Design review of the part shown in the three views and the two pictorial views. Dimensions are in mm from the part's minimum x, y and z. A direction names the side the tool comes from. Give positions to 0.01 mm unless a question says otherwise; leave off trailing zeros. Order: outer loops, then holes, each group sorted by start corner. A loop starts at its lowest first (then second) coordinate and runs counter-clockwise, first axis right, second up.
Item 1: Consider section C-C (z = 156.5). Give the boundary of the cut face in (x, y).
Item 2: Machinability: for the marked faces 1, 2 and 3, which of the approach directions +Z, -Z, +X, -X, +Y, -Y give a long, thin tool a straight path to every point of the face, cutting with its end or side? Answer none if there is none.
Item 3: For probe 1 along Z at (x, y) = (27, 58.5); probe 2 along X at (y, z) = (32.5, 111); probe 3 along Y at (x, z) = (31.5, 153.5), list the stretches that pass through material, from the lowest coordinate up.
Item 4: Consider section A-A (y = 32.25). Give the boundary of the cut face in (x, z).
Item 5: For P1, Ø8, axis at y = 23.5, z = 147.5, coming from the -X side; P2, Ø10, axis at y = 51.5, z = 87.5, coming from the -X side; P3, Ø4, axis at y = 41, z = 140, coming from the -X side, all flat-tipped, find the tip position at first contact; note any pin that passes through.
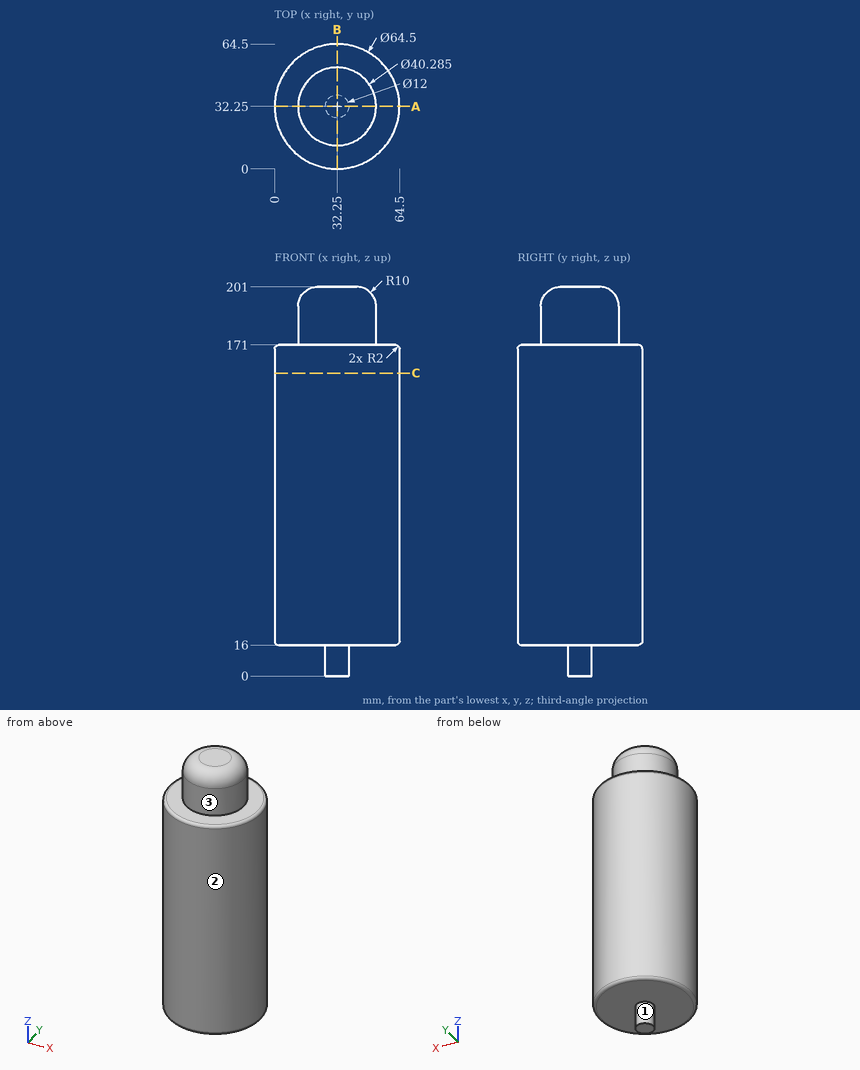
Resolved:
1. outline: circle Ø64.5 at (32.25, 32.25)
2. face 1: -Z
2. face 2: +Z, -Z
2. face 3: +Z
3. probe 1: z = 16 to 171
3. probe 2: x = 0 to 64.5
3. probe 3: y = 0.01 to 64.49
4. outline: (0, 18) arc R2 ccw to (2, 16) - (26.25, 16) - (26.25, 0) - (38.25, 0) - (38.25, 16) - (62.5, 16) arc R2 ccw to (64.5, 18) - (64.5, 169) arc R2 ccw to (62.5, 171) - (52.39, 171) - (52.39, 191) arc R10 ccw to (42.39, 201) - (22.11, 201) arc R10 ccw to (12.11, 191) - (12.11, 171) - (2, 171) arc R2 ccw to (0, 169) - close
5. P1: stops at x = 0.35
5. P2: stops at x = 3.32
5. P3: stops at x = 0.71
